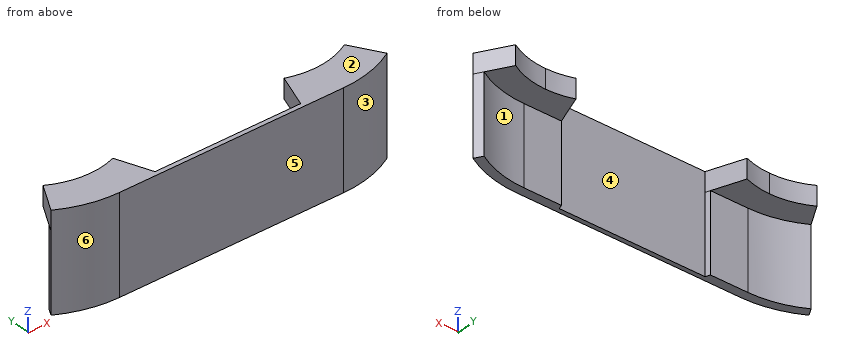
from build123d import *

# Parameters (mm, degrees)
EXTRUDE_1_DEPTH = 8.5
EXTRUDE_START   = -34.55
EXTRUDE_5_DEPTH = 34.55


with BuildPart() as part:
    # 草图1 → 凸台-拉伸1 (new body)
    with BuildSketch(Plane.XY):
        with BuildLine():
            Line((0, -50), (25, -50))
            Line((25, -50), (75, -50))
            Line((75, -50), (100, -50))
            ThreePointArc((100, -50), (112.940952255, -48.296291314), (125, -43.301270189))
            Line((125, -43.301270189), (117.25, -29.877876431))
            ThreePointArc((117.25, -29.877876431), (108.929257056, -33.324441007), (100, -34.5))
            ThreePointArc((100, -34.5), (94.00913787, -33.975867479), (88.200305055, -32.419395417))
            Line((88.200305055, -32.419395417), (82.529428755, -48))
            Line((82.529428755, -48), (75, -48))
            Line((75, -48), (25, -48))
            Line((25, -48), (17.470571245, -48))
            Line((17.470571245, -48), (11.799694945, -32.419395417))
            ThreePointArc((11.799694945, -32.419395417), (5.99086213, -33.975867479), (0, -34.5))
            ThreePointArc((0, -34.5), (-8.929257056, -33.324441007), (-17.25, -29.877876431))
            Line((-17.25, -29.877876431), (-25, -43.301270189))
            ThreePointArc((-25, -43.301270189), (-12.940952255, -48.296291314), (0, -50))
        make_face()
    extrude(amount=EXTRUDE_1_DEPTH)

    # 草图3 → 凸台-拉伸5 (add)
    with BuildSketch(Plane.XY.offset(EXTRUDE_START)):
        with BuildLine():
            Line((-23, -39.837168574), (-25, -43.301270189))
            ThreePointArc((-25, -43.301270189), (-12.940952255, -48.296291314), (0, -50))
            Line((0, -50), (100, -50))
            ThreePointArc((100, -50), (112.940952255, -48.296291314), (125, -43.301270189))
            Line((125, -43.301270189), (123, -39.837168574))
            ThreePointArc((123, -39.837168574), (111.905676075, -44.432588009), (100, -46))
            Line((100, -46), (83.257369224, -46))
            Line((83.257369224, -46), (82.529428755, -48))
            Line((82.529428755, -48), (17.470571245, -48))
            Line((17.470571245, -48), (16.742630776, -46))
            Line((16.742630776, -46), (0, -46))
            ThreePointArc((0, -46), (-11.905676075, -44.432588009), (-23, -39.837168574))
        make_face()
    extrude(amount=EXTRUDE_5_DEPTH)


solid = part.part
Build history of the part. All positions in model axes, mm. Face numbers are marked on the shaded views. A direction names the side the tool comes from. Give positions to 0.01 mm unless a question says otherwise; leave off trailing zeros. Order: outer loops, then holes, each group sorted by start corner. A loop starts at its lowest first (then second) coordinate and runs counter-clockwise, first axis right, second up. Notation, with made-up numbers: M 63.5,42.5 L 86.5,42.5 A27 ccw 86.5,75.5 Z; hole C 24.5,0.5 d3. An arc over 180 degrees is marked long. Use one line per item in the form item = value.
Q1. Which spindle directions (+Z, -Z, +X, -X, +Y, -Y) get a long thin tool onto all of the face, cutting with end or side? Do the marked faces 1 and 2. Say none if no direction does.
Conclusion:
face_1 = -Z, +Y
face_2 = +Z, +X, -X, +Y, -Y
Q2. Slice it at B-B, the plane z = -2.5. Write the cut outline in (x, y), and give its area (3 significant figures).
Conclusion:
outline = M -25,-43.3 A50 ccw 0,-50 L 100,-50 A50 ccw 125,-43.3 L 123,-39.84 A46 cw 100,-46 L 83.26,-46 L 82.53,-48 L 17.47,-48 L 16.74,-46 L 0,-46 A46 cw -23,-39.84 Z
area = 469 mm2
Q3. Slice it at C-C, the plane x = -3. Write the cut outline in (y, z).
Conclusion:
outline = M -49.91,-34.55 L -45.9,-34.55 L -45.9,0 L -34.37,0 L -34.37,8.5 L -49.91,8.5 Z
Q4. Slice it at A-A, the plane y = -38.5. Write the cut outline in (x, z), and give its area (3 significant figures).
Conclusion:
outline = M -22.23,0 L 14.01,0 L 14.01,8.5 L -22.23,8.5 Z; M 85.99,0 L 122.23,0 L 122.23,8.5 L 85.99,8.5 Z
area = 616 mm2
Q5. Slice it at D-D, the plane x = 40. Write the cut outline in (y, z), and give its area (3 significant figures).
Conclusion:
outline = M -50,-34.55 L -48,-34.55 L -48,8.5 L -50,8.5 Z
area = 86.1 mm2
Q6. Wall check: probe 1 along Y at (x, z) = (89, -16.5); probe 2 along Z at (x, y) = (11.5, -42); probe 3 along Y at (x, z) = (69.5, 3). Give the ranges that are in metal, low to high.
Conclusion:
probe_1 = -50 to -46
probe_2 = 0 to 8.5
probe_3 = -50 to -48
Q7. Pull direction X, two halves, no side cores. Call the marked faces 3, 4, 5 and 6: released by +X, released by -X, zero draft, split by the parting line, or undercut.
Conclusion:
face_3 = released by +X
face_4 = undercut
face_5 = zero draft
face_6 = released by -X
Q8. Pin check, flat tips, straight feed: P1, Ø8.5, axis at x = 8.5, z = -11.5, coming from the +Y side; P2, Ø12, axis at x = -7, z = -23, coming from the +Y side; P3, Ø13, axis at x = 59, z = -13.5, coming from the +Y side. Stop position of each tip, or through.
Conclusion:
P1 = -46
P2 = -44.12
P3 = -48
